```python
from build123d import *

# Parameters (mm, degrees)
SKETCH_1_W             = 140
SKETCH_1_H             = 193
EXTRUDE_1_DEPTH        = 2
SKETCH_2_R             = 1.6
CUT_EXTRUDE_1_DEPTH    = 120.231916868
EXTRUDE_2_DEPTH        = 23
CUT_EXTRUDE_2_DEPTH    = 172.584527274
FILLET_1_R             = 5
FILLET_2_R             = 10
SKETCH_5_R             = 2
CUT_EXTRUDE_3_DEPTH    = 122.808250952
FILLET_3_R             = 5
SKETCH_6_W             = 20
SKETCH_6_H             = 115
CUT_EXTRUDE_4_DEPTH    = 122.808250952
FILLET_START           = -23
FILLET_4_DEPTH         = 26
FILLET_4_2_DEPTH       = 2
SKETCH_7_W             = 90
SKETCH_7_H             = 25
CUT_EXTRUDE_5_DEPTH    = 122.413549491
EXTRUDE_5_DEPTH        = 5
FILLET_8_R             = 5
FILLET_8_OF_MIRROR_3_R = 5


with BuildPart() as part:
    # 스케치1 → 보스-돌출1 (new body)
    with BuildSketch(Plane(origin=(0, 0, 0), x_dir=(1, 0, 0), z_dir=(0, 1, 0))):
        Rectangle(SKETCH_1_W, SKETCH_1_H)
    extrude(amount=EXTRUDE_1_DEPTH)

    # 스케치2 → 컷-돌출1 (cut, through all)
    with BuildSketch(Plane(origin=(0, 2, 0), x_dir=(1, 0, 0), z_dir=(0, 1, 0))):
        with Locations(Location((-18.67, -93.5, 0), (0, 0, 270))):
            Circle(SKETCH_2_R)
        with Locations(Location((18.67, -93.5, 0), (0, 0, 270))):
            Circle(SKETCH_2_R)
        with Locations(Location((18.67, -56.16, 0), (0, 0, 270))):
            Circle(SKETCH_2_R)
        with Locations(Location((-18.67, -56.16, 0), (0, 0, 270))):
            Circle(SKETCH_2_R)
    extrude(amount=-CUT_EXTRUDE_1_DEPTH, mode=Mode.SUBTRACT)

    # 스케치3 → 보스-돌출2 (add)
    with BuildSketch(Plane(origin=(0, 0, 0), x_dir=(-1, 0, 0), z_dir=(0, -1, 0))):
        Polygon((70, -96.5), (70, -46.1), (50.3, -46.1), (50.3, -56.1), (53.3, -56.1), (53.3, -49.1), (67, -49.1), (67, -91.5), (54.7, -91.5), (54.7, -96.5), align=None)
    extrude_2 = extrude(amount=EXTRUDE_2_DEPTH)

    # 대칭 복사1: 보스-돌출2 across plane
    add(extrude_2.mirror(Plane(origin=(0, 0, 0), x_dir=(0, 0, 1), z_dir=(1, 0, 0))))

    # 스케치4 → 컷-돌출2 (cut, through all)
    with BuildSketch(Plane.ZY.offset(70)):
        with BuildLine():
            Line((54.05, -11.5), (54.05, -23))
            Line((54.05, -23), (75.8, -23))
            Line((75.8, -23), (75.8, -4.75))
            Line((75.8, -4.75), (60.8, -4.75))
            ThreePointArc((60.8, -4.75), (56.027029227, -6.727029227), (54.05, -11.5))
        make_face()
    extrude(amount=-CUT_EXTRUDE_2_DEPTH, mode=Mode.SUBTRACT)

    # 필렛1
    fillet_1_edges = [part.edges().sort_by_distance(p)[0] for p in [
        (-68.5, -4.75, 75.8),
        (68.5, -4.75, 75.8),
    ]]
    fillet(fillet_1_edges, radius=FILLET_1_R)

    # 필렛2
    fillet_2_edges = [part.edges().sort_by_distance(p)[0] for p in [
        (-60.15, 0, 46.1),
        (60.15, 0, 46.1),
    ]]
    fillet(fillet_2_edges, radius=FILLET_2_R)

    # 스케치5 → 컷-돌출3 (cut, through all)
    with BuildSketch(Plane(origin=(0, 2, 0), x_dir=(1, 0, 0), z_dir=(0, 1, 0))):
        with Locations(Location((47, -50.16, 0), (0, 0, 270))):
            Circle(SKETCH_5_R)
    extrude(amount=-CUT_EXTRUDE_3_DEPTH, mode=Mode.SUBTRACT)

    # 필렛3
    fillet_3_edges = [part.edges().sort_by_distance(p)[0] for p in [
        (70, -10.5, 96.5),
        (-70, -10.5, 96.5),
    ]]
    fillet(fillet_3_edges, radius=FILLET_3_R)

    # 스케치6 → 컷-돌출4 (cut, through all)
    with BuildSketch(Plane(origin=(0, 2, 0), x_dir=(1, 0, 0), z_dir=(0, 1, 0))):
        with Locations((-60, 39)):
            Rectangle(SKETCH_6_W, SKETCH_6_H)
        with Locations((60, 39)):
            Rectangle(SKETCH_6_W, SKETCH_6_H)
    extrude(amount=-CUT_EXTRUDE_4_DEPTH, mode=Mode.SUBTRACT)

    # 필렛4: read off the stored shape, not the designer's step
    # 필렛4 outline → 필렛4 (cut)
    with BuildSketch(Plane(origin=(0, 0, 0), x_dir=(1, 0, 0), z_dir=(0, 1, 0)).offset(FILLET_START)):
        with BuildLine():
            Line((70, -18.5), (60, -18.5))
            ThreePointArc((60, -18.5), (67.071067812, -21.428932188), (70, -28.5))
            Line((70, -28.5), (70, -18.5))
        make_face()
        with BuildLine():
            ThreePointArc((-70, -28.5), (-67.071067812, -21.428932188), (-60, -18.5))
            Line((-60, -18.5), (-70, -18.5))
            Line((-70, -18.5), (-70, -28.5))
        make_face()
    extrude(amount=FILLET_4_DEPTH, mode=Mode.SUBTRACT)

    # Fillet 4 2 outline → Fillet 4 2 (add)
    with BuildSketch(Plane(origin=(0, 0, 0), x_dir=(1, 0, 0), z_dir=(0, 1, 0))):
        with BuildLine():
            Line((50, -18.5), (60, -18.5))
            ThreePointArc((60, -18.5), (52.928932188, -15.571067812), (50, -8.5))
            Line((50, -8.5), (50, -18.5))
        make_face()
        with BuildLine():
            ThreePointArc((-50, -8.5), (-52.928932188, -15.571067812), (-60, -18.5))
            Line((-60, -18.5), (-50, -18.5))
            Line((-50, -18.5), (-50, -8.5))
        make_face()
    extrude(amount=FILLET_4_2_DEPTH)

    # 스케치7 → 컷-돌출5 (cut, through all)
    with BuildSketch(Plane.XZ):
        with Locations((0, -84)):
            Rectangle(SKETCH_7_W, SKETCH_7_H)
    extrude(amount=-CUT_EXTRUDE_5_DEPTH, mode=Mode.SUBTRACT)

    # 스케치11 → 보스-돌출5 (add)
    with BuildSketch(Plane.ZY.offset(50)):
        Polygon((-96.5, 0), (-96.5, -9.324233381), (-76.5, -13.973838302), (-76.5, 0), align=None)
    extrude_5 = extrude(amount=-EXTRUDE_5_DEPTH)

    # 필렛8
    fillet_8_edges = [part.edges().sort_by_distance(p)[0] for p in [
        (-47.5, 0, -76.5),
    ]]
    fillet(fillet_8_edges, radius=FILLET_8_R)

    # 대칭 복사3: 보스-돌출5 across plane
    add(extrude_5.mirror(Plane(origin=(0, 0, 0), x_dir=(0, 0, 1), z_dir=(1, 0, 0))))

    # 필렛8 of 대칭 복사3
    fillet_8_of_mirror_3_edges = [part.edges().sort_by_distance(p)[0] for p in [
        (47.5, 0, -76.5),
    ]]
    fillet(fillet_8_of_mirror_3_edges, radius=FILLET_8_OF_MIRROR_3_R)


solid = part.part
```
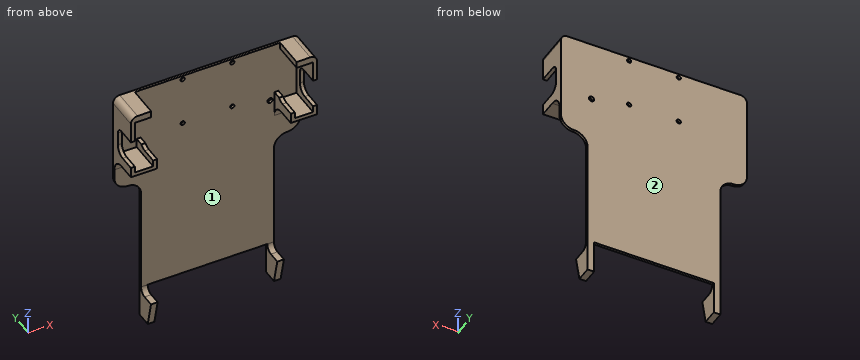
Work out the finished part from the listing and answer in its coordinate system (mm). Face numbers are marked on the shaded views. Give positions to 0.01 mm unless a question says otherwise; leave off trailing zeros. Write each loop counter-clockwise with the first axis right and the second up, starting at its lowest first coordinate (ties: lowest second). Pieces come first, ordered by that corner, then holes. Notation, with made-up numbers: (49, 63.5) -> (62, 63.5) arc R21 ccw to (62, 81.5) -> close; hole circle Ø6 at (26, 20). An arc over 180 degrees is marked (long way). Write each question's results on one line, items separated by ' | '.
1. Each of these flat-tipped pins is pushed along its axis until it touches: pin 1 Ø8 at (y, z) = (-4.5, -82.5) entering from -X; pin 2 Ø4 at (x, z) = (22.5, 72) entering from -Y; pin 3 Ø11.5 at (y, z) = (-15.5, 74.5) entering from -X; pin 4 Ø12 at (y, z) = (-8.5, -9) entering from +X. Where does it stop, or does it pass through?
Data:
pin 1: x = -50 | pin 2: y = 0 | pin 3: x = -70 | pin 4: through
2. Determine the mould class of the marked faces 1 and 2 for opening direction X: +X half, -X half, draft (parallel to the pull), parting line (faces both ways), or undercut.
Data:
face 1: undercut | face 2: draft
3. Find section A-A on y = -18. Give the number of separate pieces and of enclosed holes in the cut face, and give its area (3 significant figures).
Data:
separate pieces: 4 | enclosed holes: 0 | area: 414 mm^2
4. Straight lines are drawn through the part: L1, parallel to X at y = -8, z = 54; L2, parallel to X at y = -0.5, z = 88; L3, parallel to Y at x = -27.5, z = 68. For each, find the intervals that lie inside material, in ascending order.
Data:
L1: -70 to -67, -53.3 to -50.3, 50.3 to 53.3, 67 to 70 | L2: -70 to -67, 67 to 70 | L3: 0 to 2
5. Find section B-B on x = -47. Determine the outline of the cut face in (y, z), and give its area (3 significant figures).
Data:
outline: (-13.97, -76.5) -> (-9.32, -96.5) -> (2, -96.5) -> (2, 96.5) -> (0, 96.5) -> (0, -71.5) arc R5 cw to (-5, -76.5) -> close | area: 624 mm^2
6. Find section C-C on z = 83.5. Determine the outline of the cut face in (x, y).
Data:
outline: (-70, -23) -> (-67, -23) -> (-67, 0) -> (67, 0) -> (67, -23) -> (70, -23) -> (70, 2) -> (-70, 2) -> close
7. Find section D-D on z = -63. Determine the outline of the cut face in (x, y).
Data:
outline: (-50, 0) -> (50, 0) -> (50, 2) -> (-50, 2) -> close
